Input: part model. Units: mm. Frame: model coordinates. A direction names the side the tool comes from. Coordinates: 2 decimals unless noted, no trailing zeros. Write each loop counter-clockwise with the first axis right and the second up, starting at its lowest first coordinate (ties: lowest second). Pieces come first, ordered by that corner, then holes. Notation, with made-up numbers: M 70,41 L 86,41 A25 cw 86,61 Z; hole C 39,-13.75 d8. An arc over 180 degrees is marked long. Use one line per item in the form item = value.
Autodesk Inventor part; units mm, degrees
ref_plane "YZ Plane" through (0, 0, 0) normal (1, 0, 0) x (0, 1, 0)
ref_plane "XZ Plane" through (0, 0, 0) normal (0, 1, 0) x (-1, 0, 0)
ref_plane "XY Plane" through (0, 0, 0) normal (0, 0, 1) x (1, 0, 0)
sketch "Sketch1" plane through (0, 0, 0) normal (0, 0, 1) x (1, 0, 0)
  circle A0 centre (0, 0) radius 12.7
  dimension "d0" = 25.4
extrude "Extrusion1" add sketch "Sketch1" along normal blind 25.4
sketch "Sketch3" plane through (0, 0, 0) normal (0, 0, -1) x (-1, 0, 0)
  circle A0 centre (0, 0) radius 9.525
  dimension "d6" = 19.05
extrude "Extrusion3" cut sketch "Sketch3" against normal blind 3.175
sketch "Sketch4" plane through (0, 0, 3.175) normal (0, 0, -1) x (-1, 0, 0)
  circle A0 centre (0, 0) radius 3.683
  circle A1 centre (0, 0) radius 9.525
  arc A2 (-3.175, 8.9803) -> (3.175, 8.9803) centre (0, 0) ccw
  dimension "d40" = 7.366
extrude "Extrusion4" cut sketch "Sketch4" against normal blind 5.2926 contours A0
sketch "Sketch5" plane through (0, 0, 25.4) normal (0, 0, 1) x (1, 0, 0)
  circle A0 centre (0, 0) radius 9.525
  dimension "d13" = 19.05
extrude "Extrusion5" cut sketch "Sketch5" against normal blind 11.43
sketch "Sketch7" plane through (0, 0, 13.97) normal (0, 0, 1) x (1, 0, 0)
  circle A0 centre (0, 0) radius 3.683
  circle A1 centre (-4.7625, 0) radius 3.429
  circle A2 centre (-4.7625, 0) radius 1.6433
  circle A3 centre (0, 0) radius 4.572
  dimension "d47" = 9.144
extrude "Extrusion8" cut sketch "Sketch7" against normal blind 3.81 contours A0 A1 | A0 A1 A3 | A1 A0 A2 | A0 A2 A3 A1 | A1 A3 A2 A0 | A2 A0 | A0 A2 A3
sketch "Sketch8" plane through (0, 0, 10.16) normal (0, 0, 1) x (1, 0, 0)
  circle A0 centre (0, 0) radius 2.754
extrude "Extrusion9" cut sketch "Sketch8" against normal through all
sketch "Sketch9" plane through (0, 0, 13.97) normal (0, 0, 1) x (1, 0, 0)
  circle A0 centre (0, -6.985) radius 2.286
  circle A1 centre (0, 6.985) radius 2.286
  circle A2 centre (0, 0) radius 9.525
  line L0 (-2.1601, -6.2369) -> (-3.1173, -9.0005)
  line L1 (-2.1601, 6.2369) -> (-3.1173, 9.0005)
  line L2 (3.1173, -9.0005) -> (2.1601, -6.2369)
  line L3 (2.1601, 6.2369) -> (3.1173, 9.0005)
extrude "Extrusion10" add sketch "Sketch9" along normal blind 8.255 contours A0 | A0 L2 A2 L0 | A2 L3 A1 L1 | A1
sketch "Sketch10" plane through (0, 0, 22.225) normal (0, 0, 1) x (1, 0, 0)
  circle A0 centre (0, -6.985) radius 1.27
  circle A1 centre (0, 6.985) radius 1.27
  circle A2 centre (0, -6.985) radius 2.286
  circle A3 centre (0, 6.985) radius 2.286
  point P0 (0, 0)
  dimension "d28" = 2.54
  dimension "d29" = 2.54
extrude "Extrusion11" cut sketch "Sketch10" against normal blind 7.62 contours A0 | A1
chamfer "Chamfer1" distance 6.35 angle 15 1 edges at (-12.7, 0, 0) measured on face at (12.6588, -1.0219, 16.9333)
sketch "Sketch12" plane through (0, 0, 3.175) normal (0, 0, -1) x (-1, 0, 0)
  circle A0 centre (5.9436, 0) radius 1.27
  circle A1 centre (-5.9436, 0) radius 1.27
  point P0 (0, 0)
  dimension "d41" = 2.54
  dimension "d42" = 2.54
  dimension "d43" = 5.9436
  dimension "d44" = 5.9436
extrude "Extrusion13" cut sketch "Sketch12" against normal blind 6.35
properties part number "Cap no LED"
(1) Section query C-C on z = 12. Return the cut outline in (x, y), plus the area to 3 significant figures.
Computed:
outline = C 0,0 d25.4; hole C 0,0 d9.14
area = 441 mm^2
(2) First-contact query: pin 1 Ø2.5 at (x, y) = (-0.5, 7) entering from +Z (3 decimals); pin 2 Ø9.5 at (x, y) = (1.5, -3.5) entering from -Z (3 decimals); pin 3 Ø0.8 at (x, y) = (6, -0.5) entering from -Z (3 decimals). Flat tips, straight axial feed; report the tip coordinate or a pass-through.
Computed:
pin_1 = 22.225
pin_2 = 3.175
pin_3 = 9.525
(3) Line query: probe 1 along Y at (x, z) = (0, 18.5) (3 decimals); probe 2 along Y at (x, z) = (0, 13.2); probe 3 along Y at (x, z) = (0, 8.85). Output: solid intervals per line, ascending.
Computed:
probe_1 = -12.7 to -8.255, -5.715 to -4.699, 4.699 to 5.715, 8.255 to 12.7
probe_2 = -12.7 to -4.57, 4.57 to 12.7
probe_3 = -12.7 to -2.75, 2.75 to 12.7
(4) Pull-direction query (X, two-part tool) for faces 1 (the flat face through (0, 10, 0)), 2 (the flat face through (2.645, -7.638, 18.04)), 3 (the conical face through (5.97, 9.364, 0.397)), 4 (the cylindrical face through (6.951, -0.773, 6.306)); classes: pulls with the +X half, pulls with the -X half, needs draft (parallel to the pull), parting line crosses it, or undercut.
Computed:
face_1 = needs draft
face_2 = undercut
face_3 = parting line crosses it
face_4 = undercut
(5) Set-up query: faces 5 (the cylindrical face through (-2.185, -1.676, 9.326)), 6 (the flat face through (-4.4, 2.1, 13.97)), 7 (the cylindrical face through (-4.936, -0.773, 6.306)). Return all of +Z, -Z, +X, -X, +Y, -Y with unobstructed straight access to the full face (end or side cutting, diameter ignored); none if empty.
Computed:
face_5 = +Z, -Z
face_6 = +Z
face_7 = -Z
(6) Section query B-B on z = 19. State how many separate pieces and enclosed holes the cut face has, plus the area to 3 significant figures.
Computed:
separate_pieces = 1
enclosed_holes = 3
area = 255 mm^2
(7) Section query D-D on z = 7.75. Return the cut outline in (x, y), plus the area to 3 significant figures.
Computed:
outline = C 0,0 d25.4; hole C -5.94,0 d2.54; hole C 0,0 d7.37; hole C 5.94,0 d2.54
area = 454 mm^2
